Can you work these out from the drawing? Everything is in mm from the part's minimum corner. Give positions to 0.01 mm unless a question says otherwise; leave off trailing zeros. Loops run counter-clockwise (first coordinate to the right, second up) from the corner with the lowest first, then second, coordinate; pieces in that order, holes last. Notation, with made-up numbers: M -18.75,81.25 L 7.25,81.25 A27 ccw 7.25,103.25 Z; hole C 10,26 d8. An arc over 180 degrees is marked long. Use CSV: the item, a comma, the result in double quotes.
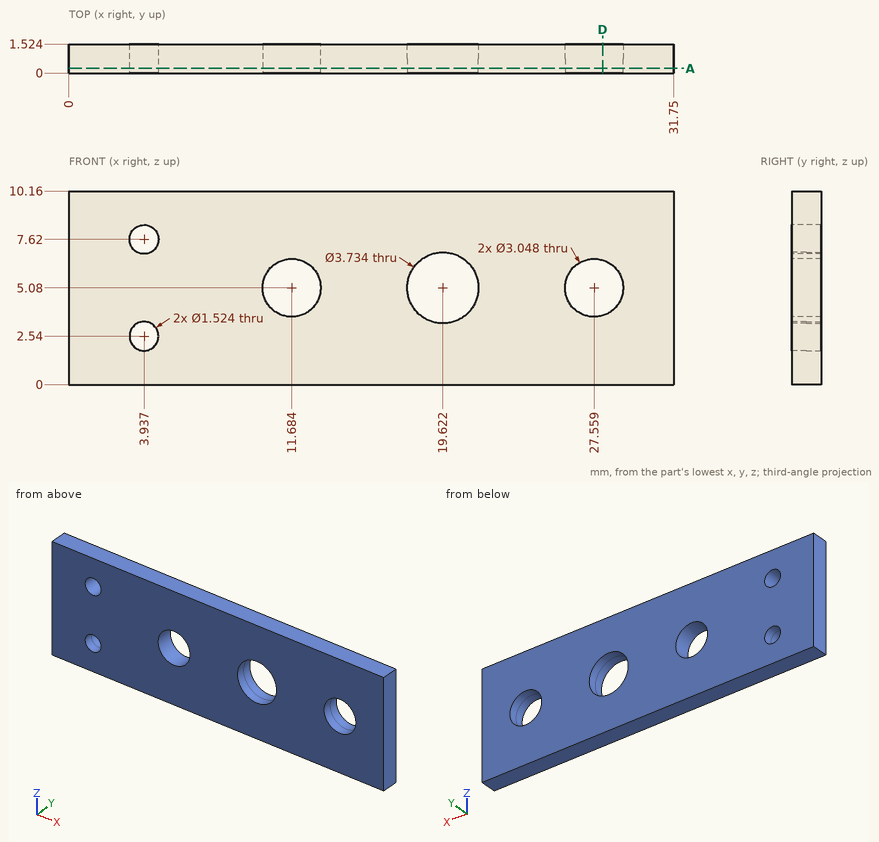
Q1. Please list where these lines run through material, in increasing order: L1, parallel to Z at x = 3.5, y = 0.3 (1 decimal); L2, parallel to Z at x = 19.5, y = 0.45; L3, parallel to Z at x = 19, y = 1.2. Write a range as from..to.
Model answer:
L1,"0..1.9, 3.2..7, 8.2..10.2"
L2,"0..3.22, 6.94..10.16"
L3,"0..3.32, 6.84..10.16"
Q2. I want a section at D-D, the plane x = 28. Please give me the cut outline in (y, z) (1 decimal).
Model answer:
outline,"M 0,0 L 1.5,0 L 1.5,3.6 L 0,3.6 Z; M 0,6.5 L 1.5,6.5 L 1.5,10.2 L 0,10.2 Z"
Q3. I want a section at A-A, the plane y = 0.25. State how many separate pieces and enclosed holes the cut face has.
Model answer:
separate pieces,"1"
enclosed holes,"5"
